from build123d import *

# Parameters (mm, degrees)
F1_DEPTH     = 2
F3_DEPTH     = 15
F4_W         = 15
F4_H         = 36.1711822092
F5_DEPTH     = 2
F6_W         = 16
F6_H         = 2
F7_DEPTH     = 15
F8_R         = 2
F11_DEPTH    = 10
F12_R        = 2.25
F13_DEPTH    = 25
F14_T1_DEPTH = 10


# Not quite as in the source:
# - a fillet or chamfer that OpenCascade refuses, or shapes differently, is made with other operations: its cross-section is extruded or revolved along the edge and cut away or added


with BuildPart() as f1:
    # F0 (on Top) → F1 (new body)
    with BuildSketch(Plane.XY):
        with BuildLine():
            Line((-7.5, 60), (-7.5, 0))
            Line((-7.5, 0), (7.5, 0))
            Line((7.5, 0), (7.5, 60))
            ThreePointArc((7.5, 60), (0, 67.5), (-7.5, 60))
        make_face()
    extrude(amount=F1_DEPTH)

    # F2 (on face) → F3 (join, through all)
    with BuildSketch(Plane.YZ.offset(7.5)):
        with BuildLine():
            Line((-9.1977466834, 9.85), (-1.5320888862, 0.7144247806))
            ThreePointArc((-1.5320888862, 0.7144247806), (-0.8452365235, 0.1873844259), (0, 0))
            Line((0, 0), (0, 2))
            Line((0, 2), (-7.6656577972, 11.1355752194))
            ThreePointArc((-7.6656577972, 11.1355752194), (-8.3525101599, 11.6626155741), (-9.1977466834, 11.85))
            Line((-9.1977466834, 11.85), (-9.1977466834, 9.85))
        make_face()
    extrude(amount=-F3_DEPTH)

    # F6 (on face) → F7 (join, through all)
    with BuildSketch(Plane(origin=(-7.5, 0, 0), x_dir=(0, -1, 0), z_dir=(-1, 0, 0))):
        with Locations((17.1977466834, 10.85)):
            Rectangle(F6_W, F6_H)
    extrude(amount=-F7_DEPTH)

    # F8
    f8_edges = [f1.edges().sort_by_distance(p)[0] for p in [
        (0, 0, 0),
        (0, 0, 2),
        (0, -9.197747, 11.85),
        (0, -9.197747, 9.85),
    ]]
    fillet(f8_edges, radius=F8_R)

    # F10 (on face) → F11 (join)
    with BuildSketch(Plane.XZ.offset(25.1977466834)):
        with BuildLine():
            Line((-7.5, 9.85), (7.5, 9.85))
            Line((7.5, 9.85), (15.3476885433, 5.319134907))
            Line((15.3476885433, 5.319134907), (16.3476885433, 7.0511857146))
            Line((16.3476885433, 7.0511857146), (8.384588029, 11.6486839401))
            ThreePointArc((8.384588029, 11.6486839401), (7.9574981533, 11.8161493535), (7.5, 11.85))
            Line((7.5, 11.85), (-7.5, 11.85))
            Line((-7.5, 11.85), (-7.5, 9.85))
        make_face()
    extrude(amount=F11_DEPTH)

    # F12 (on face) → F13 (cut)
    with BuildSketch(Plane.XY.offset(2)):
        with Locations((0, 60)):
            Circle(F12_R)
        with Locations((0, 30)):
            Circle(F12_R)
    extrude(amount=-F13_DEPTH, mode=Mode.SUBTRACT)

    # F14: fillet of radius 2 on 1 edges, made by hand

    # F14_s2 → F14_t1 (join)
    with BuildSketch(Plane.XZ.offset(25.1977466834)):
        with BuildLine():
            ThreePointArc((6.9641016151, 9.85), (7.4817397053, 9.7818516526), (7.9641016151, 9.5820508076))
            Line((7.9641016151, 9.5820508076), (7.5, 9.85))
            Line((7.5, 9.85), (6.9641016151, 9.85))
        make_face()
    extrude(amount=F14_T1_DEPTH)


with BuildPart() as f5:
    # F4 (on face) → F5 (new body)
    with BuildSketch(Plane.XY.offset(2)):
        with Locations((0, -25.7512489018)):
            Rectangle(F4_W, F4_H)
    extrude(amount=F5_DEPTH)


solid = f1.part
Can you work these out from the model? Positions are in its coordinate system, mm. A direction names the side the tool comes from. Round coordinates to 2 decimals unless told otherwise and drop trailing zeros. Write each loop counter-clockwise with the first axis right and the second up, starting at its lowest first coordinate (ties: lowest second). Pieces come first, ordered by that corner, then holes. Notation, with made-up numbers: (-28, -20.75) - (-12, -20.75) arc R13 ccw to (-12, 4.25) - close; hole circle Ø9 at (1.25, 35). An arc over 180 degrees is marked (long way). Write each question's results on one line, items separated by ' | '. Start each with the question number.
1) We'd pull the mould along Y, two halves only. Please class faces 4 (the flat face through (0, -22, 11.85)), 5 (the cylindrical face through (0.16, 67.5, 0.99)), 6 (the cylindrical face through (-0.488, 27.804, 1.014)): released by +Y, released by -Y, zero draft, split by the parting line, or undercut.
2) Which directions (+Z, -Z, +X, -X, +Y, -Y) give clear straight access to the entire face, cutting with the end or side of a thin tool? Please do faces 1 (the flat face through (-7.5, 9.1, 1.6)), 2 (the flat face through (7.5, 14.4, 1.6)), 3 (the flat face through (0, 35, 2)).
3) Suppose I cut it at D-D (y = -17.5). List the corners of the cut face in (x, z) for me.
4) Please list where these lines run through material, in increasing order: line 1 (Y direction, x = 0, z = 1.25); line 2 (Z direction, x = -5.75, y = -29); line 3 (Z direction, x = 5, y = 32.5).
5) For pin 1 Ø12 at (x, y) = (-3, 23) entering from +Z; pin 2 Ø1 at (x, z) = (-5, 2) entering from -Y; pin 3 Ø4.5 at (x, y) = (-3, -25) entering from -Z; pin 4 Ø5 at (x, y) = (11.5, 51) entering from -Z, each with a flat end and sliding along its axis, tell me the tip position at first contact or that it passes through.
6) Suppose I cut it at C-C (z = 8). List the corners of the cut face in (x, y) for me.
7) Suppose I cut it at B-B (x = 0). List the corners of the cut face in (y, z) for me, and give its area (3 significant figures).
8) Suppose I cut it at A-A (y = 30). List the corners of the cut face in (x, z) for me, and give its area (3 significant figures).
Here are the results:
1) face 4: zero draft | face 5: released by +Y | face 6: undercut
2) face 1: +Z, -Z, -X, +Y, -Y | face 2: +Z, -Z, +X, +Y | face 3: +Z, +X, -X, +Y
3) outline: (-7.5, 9.85) - (7.5, 9.85) - (7.5, 11.85) - (-7.5, 11.85) - close
4) line 1: y = -1.98 to 27.75, 32.25 to 57.75, 62.25 to 67.5 | line 2: z = 9.85 to 11.85 | line 3: z = 0 to 2
5) pin 1: stops at z = 2 | pin 2: stops at y = -3.03 | pin 3: stops at z = 9.85 | pin 4: passes through
6) outline: (-7.5, -7.65) - (7.5, -7.65) - (7.5, -5.03) - (-7.5, -5.03) - close; (10.7, -35.2) - (14.7, -35.2) - (14.7, -25.2) - (10.7, -25.2) - close
7) outline: (-35.2, 9.85) - (-10.13, 9.85) arc R2 cw to (-8.6, 9.14) - (-1.53, 0.71) arc R2 ccw to (0, 0) - (27.75, 0) - (27.75, 2) - (0.93, 2) arc R2 cw to (-0.6, 2.71) - (-7.67, 11.14) arc R2 ccw to (-9.2, 11.85) - (-35.2, 11.85) - close; (32.25, 0) - (57.75, 0) - (57.75, 2) - (32.25, 2) - close; (62.25, 0) - (67.5, 0) - (67.5, 2) - (62.25, 2) - close | area: 197 mm2
8) outline: (-7.5, 0) - (-2.25, 0) - (-2.25, 2) - (-7.5, 2) - close; (2.25, 0) - (7.5, 0) - (7.5, 2) - (2.25, 2) - close | area: 21.0 mm2
